```python
from build123d import *
from OCP.BRepFilletAPI import BRepFilletAPI_MakeChamfer

# Parameters (mm, degrees)
BOSS_EXTRUDE1_DEPTH = 40
CHAMFER1_SIZE       = 1
CHAMFER1_SIZE2      = 0.732050808


with BuildPart() as part:
    # Sketch1 → Boss-Extrude1 (new body)
    with BuildSketch(Plane.XY):
        Polygon((0, 11.745081595), (-10.171539031, -5.872540798), (10.171539031, -5.872540798), align=None)
        Polygon((0, 7.745081595), (-6.707437416, -3.872540798), (6.707437416, -3.872540798), align=None, mode=Mode.SUBTRACT)
    extrude(amount=BOSS_EXTRUDE1_DEPTH)

    # Chamfer1: one chamfer whose edges measure the first distance from different faces: ONE call of the kernel's chamfer builder (chamfer() names one face for all edges)
    chamfer1_edges_1 = [part.edges().sort_by_distance(p)[0] for p in [
        (10.171539031, -5.872540798, 20),
    ]]
    chamfer1_side_1 = [part.faces().sort_by_distance(p)[0] for p in [
        (0, -5.872540798, 20),
    ]]
    chamfer1_edges_2 = [part.edges().sort_by_distance(p)[0] for p in [
        (-10.171539031, -5.872540798, 20),
    ]]
    chamfer1_side_2 = [part.faces().sort_by_distance(p)[0] for p in [
        (-5.085769515, 2.936270399, 20),
    ]]
    chamfer1_edges_3 = [part.edges().sort_by_distance(p)[0] for p in [
        (0, 11.745081595, 20),
    ]]
    chamfer1_side_3 = [part.faces().sort_by_distance(p)[0] for p in [
        (5.085769515, 2.936270399, 20),
    ]]
    chamfer1 = BRepFilletAPI_MakeChamfer(part.part.solid().wrapped)
    for e in chamfer1_edges_1:
        chamfer1.Add(CHAMFER1_SIZE, CHAMFER1_SIZE2, e.wrapped, chamfer1_side_1[0].wrapped)  # the first distance lies on this face
    for e in chamfer1_edges_2:
        chamfer1.Add(CHAMFER1_SIZE, CHAMFER1_SIZE2, e.wrapped, chamfer1_side_2[0].wrapped)  # the first distance lies on this face
    for e in chamfer1_edges_3:
        chamfer1.Add(CHAMFER1_SIZE, CHAMFER1_SIZE2, e.wrapped, chamfer1_side_3[0].wrapped)  # the first distance lies on this face
    add(Compound.cast(chamfer1.Shape()), mode=Mode.REPLACE)


solid = part.part
```
Verification items for the finished model (mm, model axes). A direction names the side the tool comes from. Coordinates: 2 decimals unless noted, no trailing zeros. Write each loop counter-clockwise with the first axis right and the second up, starting at its lowest first coordinate (ties: lowest second). Pieces come first, ordered by that corner, then holes. Notation, with made-up numbers: M 36.5,19 L 52.5,19 A11 ccw 52.5,25 Z; hole C 88,47 d11. An arc over 180 degrees is marked long. One line per item, written item: value.
Item 1: Mould release check, pull along Y, two halves, no side actions. Record for faces 1 (the flat face through (-4.95, 3.17, 19.72)), 2 (the flat face through (3.401, 1.855, 19.72)), 3 (the flat face through (0, -5.873, 20)): pulls with the +Y half, pulls with the -Y half, needs draft (parallel to the pull), parting line crosses it, or undercut.
Check sheet entries:
face 1: pulls with the +Y half
face 2: undercut
face 3: pulls with the -Y half
Item 2: Section check D-D, the plane x = 7.75. Record the boundary of the cut face in (y, z).
Check sheet entries:
outline: M -5.87,0 L -1.68,0 L -1.68,40 L -5.87,40 Z
Item 3: Scan lines: line 1 along X through (y, z) = (1.5, 12.5) (3 decimals); line 2 along Y through (x, z) = (6.5, 28.5); line 3 along X through (y, z) = (-3.5, 22). Record each from-to range of solid material in increasing order.
Check sheet entries:
line 1: x = -5.915 to -3.606, 3.606 to 5.915
line 2: y = -5.87 to -3.87, -3.51 to 0.49
line 3: x = -8.8 to -6.49, 6.49 to 8.8
Item 4: Gauge pin test, flat ends, axial feed: pin 1 Ø4 at (y, z) = (3.5, 31) entering from -X (3 decimals); pin 2 Ø1.5 at (x, y) = (1, 4) entering from -Z; pin 3 Ø6.5 at (x, z) = (-2, 26) entering from +Y; pin 4 Ø5 at (y, z) = (9, 6) entering from -X. Record the tip position at first contact, or that the pin passes through.
Check sheet entries:
pin 1: stops at x = -5.915
pin 2: passes through
pin 3: stops at y = 11.11
pin 4: stops at x = -3.03
Item 5: Section check A-A, the plane z = 16. Record the boundary of the cut face in (x, y), plus the area to 3 significant figures.
Check sheet entries:
outline: M -9.67,-5.01 L -9.44,-5.87 L 9.17,-5.87 L 9.81,-5.24 L 0.5,10.88 L -0.37,11.11 Z; hole M -6.71,-3.87 L 6.71,-3.87 L 0,7.75 Z
area: 100 mm^2
Item 6: Access from +Z, -Z, +X, -X, +Y, -Y to the whole of each face (thin tool, end or side, straight path). Record for faces 4 (the flat face through (-3.307, 2.018, 19.72)), 5 (the flat face through (-9.554, -5.446, 19.72)).
Check sheet entries:
face 4: +Z, -Z
face 5: +Z, -Z, -X, -Y
Item 7: Section check C-C, the plane x = -2. Record the boundary of the cut face in (y, z).
Check sheet entries:
outline: M -5.87,0 L -3.87,0 L -3.87,40 L -5.87,40 Z; M 4.28,0 L 8.28,0 L 8.28,40 L 4.28,40 Z
Item 8: Section check B-B, the plane y = 4.5. Record the boundary of the cut face in (x, z), plus the area to 3 significant figures.
Check sheet entries:
outline: M -4.18,0 L -1.87,0 L -1.87,40 L -4.18,40 Z; M 1.87,0 L 4.18,0 L 4.18,40 L 1.87,40 Z
area: 185 mm^2
